Read the model definition and answer for the solid it produces. Units are mm, in the model's axes. Face numbers are marked on the shaded views. A direction names the side the tool comes from. Give positions to 0.01 mm unless a question says otherwise; leave off trailing zeros. Order: outer loops, then holes, each group sorted by start corner. A loop starts at its lowest first (then second) coordinate and runs counter-clockwise, first axis right, second up.
Item 1: A cutting plane is placed at D-D (x = 4). Write down the section's boundary in (y, z), plus the area to 3 significant figures.
Item 2: The mould has two halves that part along X. Classify the marked faces 3 and 4: +X half, -X half, draft (parallel to the pull), parting line (faces both ways), or undercut.
Item 3: A cutting plane is placed at A-A (z = 0). Write down the section's boundary in (x, y) (3 decimals).
Item 4: Given pin 1 Ø7 at (y, z) = (104, 0) entering from -X; pin 2 Ø5 at (y, z) = (72.5, 7) entering from -X; pin 3 Ø1 at (x, y) = (-2, 73.5) entering from -Z, each flat-ended and moving along its own axis, determine where each tip first touches the part or whether it passes through.
Item 5: A cutting plane is placed at B-B (x = 0). Write down the section's boundary in (y, z) (3 decimals), plus the area to 3 significant figures.
Item 6: A cutting plane is placed at C-C (y = 66.5). Write down the section's boundary in (x, z), plus the area to 3 significant figures.
Item 7: Which of the six approach directions +Z, -Z, +X, -X, +Y, -Y give full straight-line access (tool end or side, diameter ignored) to the marked faces 1 and 2?
Item 8: Find the intervals of material crossed by line 1 along Y through (x, z) = (-3.25, 0); line 2 along Z through (x, y) = (0, 104); line 3 along Z through (x, y) = (-1.25, 104), in increasing order.
from build123d import *

# Parameters (mm, degrees)
SKETCH5_R                           = 9.525
BOSS_EXTRUDE4_DEPTH                 = 30
SKETCH6_R                           = 6
BOSS_EXTRUDE6_DEPTH                 = 110
CUT_EXTRUDE1_REACH                  = 112.822
CUT_EXTRUDE1_END_RADIUS             = 6
SKETCH7_R                           = 3
CUT_EXTRUDE1_DIRECTION_2_REACH      = 112.822
CUT_EXTRUDE1_DIRECTION_2_END_RADIUS = 6


with BuildPart() as part:
    # Sketch5 → Boss-Extrude4 (new body)
    with BuildSketch(Plane(origin=(0, 0, 0), x_dir=(1, 0, 0), z_dir=(0, 1, 0))):
        with Locations(Location((0, 0, 0), (0, 0, 270))):
            Circle(SKETCH5_R)
    extrude(amount=BOSS_EXTRUDE4_DEPTH)

    # Sketch6 → Boss-Extrude6 (add)
    with BuildSketch(Plane(origin=(0, 0, 0), x_dir=(1, 0, 0), z_dir=(0, 1, 0))):
        with Locations(Location((0, 0, 0), (0, 0, 270))):
            Circle(SKETCH6_R)
    extrude(amount=BOSS_EXTRUDE6_DEPTH)

    # Cut-Extrude1: up to this cylinder (the profile starts inside it)
    cut_extrude1_end = Plane(origin=(0, 104, 0), z_dir=(0, -1, 0)) * Cylinder(CUT_EXTRUDE1_END_RADIUS, 238.644, mode=Mode.PRIVATE)
    # Sketch7 → Cut-Extrude1 (cut, up to the surface)
    with BuildSketch(Plane(origin=(0, 0, 0), x_dir=(0, 0, -1), z_dir=(1, 0, 0)), mode=Mode.PRIVATE) as cut_extrude1_sk1:
        with Locations(Location((0, 104, 0), (0, 0, 180))):
            Circle(SKETCH7_R)
    cut_extrude1_tool1 = extrude(cut_extrude1_sk1.sketch, amount=-CUT_EXTRUDE1_REACH, mode=Mode.PRIVATE) & cut_extrude1_end
    add(cut_extrude1_tool1.solids().sort_by_distance((0, 104, 0))[0], mode=Mode.SUBTRACT)

    # Cut-Extrude1 direction 2: up to this cylinder (the profile starts inside it)
    cut_extrude1_direction_2_end = Plane(origin=(0, 104, 0), z_dir=(0, -1, 0)) * Cylinder(CUT_EXTRUDE1_DIRECTION_2_END_RADIUS, 238.644, mode=Mode.PRIVATE)
    # Sketch7 → Cut-Extrude1 direction 2 (cut, up to the surface)
    with BuildSketch(Plane(origin=(0, 0, 0), x_dir=(0, 0, -1), z_dir=(1, 0, 0)), mode=Mode.PRIVATE) as cut_extrude1_direction_2_sk1:
        with Locations(Location((0, 104, 0), (0, 0, 180))):
            Circle(SKETCH7_R)
    cut_extrude1_direction_2_tool1 = extrude(cut_extrude1_direction_2_sk1.sketch, amount=CUT_EXTRUDE1_DIRECTION_2_REACH, mode=Mode.PRIVATE) & cut_extrude1_direction_2_end
    add(cut_extrude1_direction_2_tool1.solids().sort_by_distance((0, 104, 0))[0], mode=Mode.SUBTRACT)


solid = part.part
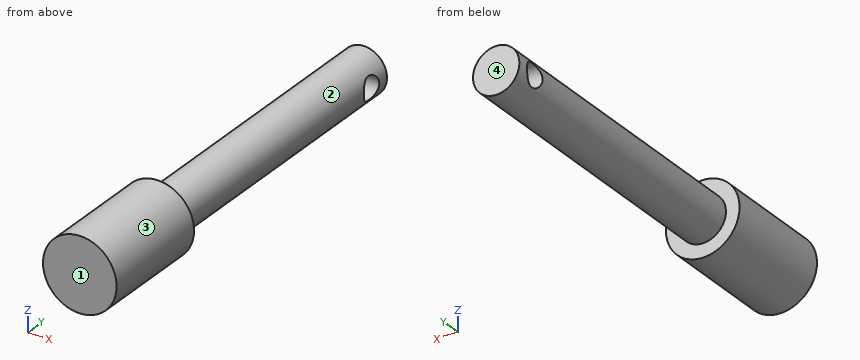
Response values:
1. outline: (0, -8.64) - (30, -8.64) - (30, -4.47) - (110, -4.47) - (110, 4.47) - (30, 4.47) - (30, 8.64) - (0, 8.64) - close; hole circle Ø6 at (104, 0)
1. area: 1,210 mm2
2. face 3: parting line
2. face 4: draft
3. outline: (-9.525, 0) - (9.525, 0) - (9.525, 30) - (6, 30) - (6, 101) - (-6, 101) - (-6, 30) - (-9.525, 30) - close; (-6, 107) - (6, 107) - (6, 110) - (-6, 110) - close
4. pin 1: stops at x = -6
4. pin 2: stops at x = -3.97
4. pin 3: stops at z = -5.81
5. outline: (0, -9.525) - (30, -9.525) - (30, -6) - (110, -6) - (110, 6) - (30, 6) - (30, 9.525) - (0, 9.525) - close; hole circle Ø6 at (104, 0)
5. area: 1,500 mm2
6. outline: circle Ø12 at (0, 0)
6. area: 113 mm2
7. face 1: +Z, -Z, +X, -X, -Y
7. face 2: +Y
8. line 1: y = 0 to 101, 107 to 110
8. line 2: z = -6 to -3, 3 to 6
8. line 3: z = -5.87 to -3, 3 to 5.87
